```python
from build123d import *

# Parameters (mm, degrees)
F0_R          = 1.75
F1_DEPTH      = 5
F2_DEPTH      = 4
F2_DEPTH_BACK = 5
F3_T1_DEPTH   = 35.3628033386
F4_R          = 11.3728971787


# Not quite as in the source:
# - a fillet or chamfer that OpenCascade refuses, or shapes differently, is made with other operations: its cross-section is extruded or revolved along the edge and cut away or added


with BuildPart() as f1:
    # F0 (on Top) → F1 (new body)
    with BuildSketch(Plane.XY):
        with BuildLine():
            ThreePointArc((-2.5631937321, 5.253964594), (1.7029722297, 5.2256762725), (3.8442630819, 8.9156418184))
            ThreePointArc((3.8442630819, 8.9156418184), (-0.4057369181, 13.1656418184), (-4.6557369181, 8.9156418184))
            ThreePointArc((-4.6557369181, 8.9156418184), (-4.095702464, 6.8069326705), (-2.5631937321, 5.253964594))
        make_face()
        with Locations((-0.4057369181, 8.9156418184)):
            Circle(F0_R, mode=Mode.SUBTRACT)
        with BuildLine():
            ThreePointArc((-2.5631937321, 5.253964594), (-4.095702464, 6.8069326705), (-4.6557369181, 8.9156418184))
            Line((-4.6557369181, 8.9156418184), (-24.6422081436, -13.4571310977))
            Line((-24.6422081436, -13.4571310977), (-21.6591717548, -16.1219939277))
            Line((-21.6591717548, -16.1219939277), (-2.5631937321, 5.253964594))
        make_face()
        Polygon((-21.6591717548, -16.1219939277), (-24.6422081436, -13.4571310977), (-24.6422081436, -16.1219939277), (-24.6422081436, -16.3715779781), align=None)
    extrude(amount=F1_DEPTH)

    # F0 (on Top) → F2 (join, two sides)
    with BuildSketch(Plane.XY) as f2_sk:
        with Locations((-0.4057369181, 8.9156418184)):
            Circle(F0_R)
    extrude(amount=-F2_DEPTH)
    extrude(f2_sk.sketch, amount=F2_DEPTH_BACK)

    # F3: fillet of radius 18.4809579153 on 1 edges, made by hand

    # F3_s2 → F3_t1 (cut)
    with BuildSketch(Plane.XY.offset(-15.1814016693)):
        with BuildLine():
            ThreePointArc((-20.5965728419, -8.9284637364), (-23.0516277567, -12.4150823252), (-24.6422081436, -16.3715779781))
            Line((-24.6422081436, -16.3715779781), (-24.6422081436, -13.4571310977))
            Line((-24.6422081436, -13.4571310977), (-20.5965728419, -8.9284637364))
        make_face()
    extrude(amount=F3_T1_DEPTH, mode=Mode.SUBTRACT)

    # F4
    f4_edges = [f1.edges().sort_by_distance(p)[0] for p in [
        (-2.563194, 5.253965, 2.5),
        (-4.655737, 8.915642, 2.5),
    ]]
    fillet(f4_edges, radius=F4_R)


solid = f1.part
```
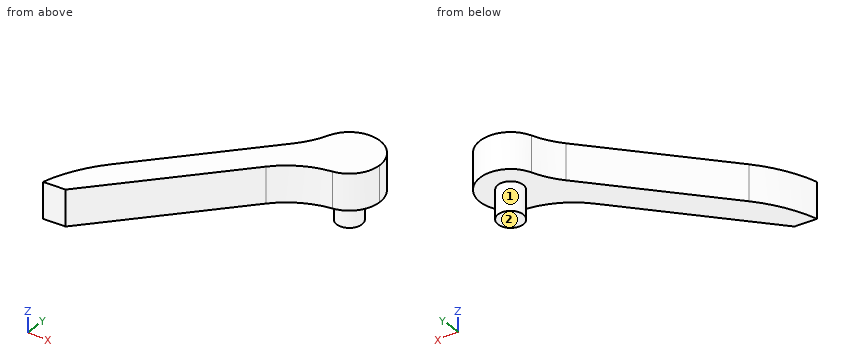
Geometry: final body of the model. Coordinates: model frame, mm. Face numbers are marked on the shaded views. A direction names the side the tool comes from. Give positions to 0.01 mm unless a question says otherwise; leave off trailing zeros. Loops run counter-clockwise (first coordinate to the right, second up) from the corner with the lowest first, then second, coordinate; pieces in that order, holes last. Notation, with made-up numbers: (41.5, 7.25) -> (95.5, 7.25) arc R24 cw to (95.5, 43.25) -> close; hole circle Ø10 at (-7.5, 38.5). An arc over 180 degrees is marked (long way). Use one line per item in the form item = value.
Item 1: Section query C-C on x = 2. Output: boundary loops of the cut face in (y, z), and give its area (3 significant figures).
A:
outline = (5.41, 0) -> (12.42, 0) -> (12.42, 5) -> (5.41, 5) -> close
area = 35.0 mm^2
Item 2: Section query A-A on z = 4. Output: boundary loops of the cut face in (x, y) (3 decimals), and give its area (3 significant figures).
A:
outline = (-24.642, -16.372) -> (-21.659, -16.122) -> (-6.285, 1.088) arc R11.373 cw to (0.302, 4.725) arc R4.25 ccw (long way) to (-4.391, 10.393) arc R11.373 cw to (-6.573, 6.77) -> (-20.597, -8.928) arc R18.481 ccw to start
area = 177 mm^2
Item 3: Access query for the marked faces 1 and 2. Directions: +Z, -Z, +X, -X, +Y, -Y. A direction counts if a zero-diameter tool reaches every point of the face in a straight line with its end or side. Return the directions, or none.
A:
face_1 = -Z
face_2 = -Z, +X, -X, +Y, -Y
Item 4: Line query: probe 1 along Z at (x, y) = (-14.25, -4.5); probe 2 along Y at (x, z) = (-2, 1); probe 3 along X at (y, z) = (-1.75, 2.25). Output: solid intervals per line, ascending.
A:
probe_1 = 0 to 5
probe_2 = 4.08 to 12.86
probe_3 = -14.18 to -8.82
Item 5: Section query D-D on z = -3.5. Output: boundary loops of the cut face in (x, y).
A:
outline = circle Ø3.5 at (-0.41, 8.92)
Item 6: Section query B-B on y = 10. Output: boundary loops of the cut face in (x, z), and give its area (3 significant figures).
A:
outline = (-4.54, 0) -> (-1.78, 0) -> (-1.78, -4) -> (0.97, -4) -> (0.97, 0) -> (3.7, 0) -> (3.7, 5) -> (-4.54, 5) -> close
area = 52.2 mm^2
